Verification items for the finished model (mm, model axes). A direction names the side the tool comes from. Round coordinates to 2 decimals unless told otherwise and drop trailing zeros. Write each loop counter-clockwise with the first axis right and the second up, starting at its lowest first coordinate (ties: lowest second). Pieces come first, ordered by that corner, then holes.
from build123d import *

# Parameters (mm, degrees)
BOSS_EXTRUDE1_DEPTH = 3
BOSS_EXTRUDE2_DEPTH = 13
SKETCH4_W           = 2.5
SKETCH4_H           = 1.5
BOSS_EXTRUDE3_DEPTH = 13
SKETCH5_R           = 1.5
CUT_EXTRUDE2_DEPTH  = 10
SKETCH6_W           = 6
SKETCH6_H           = 1.5
CUT_EXTRUDE3_DEPTH  = 10


with BuildPart() as part:
    # Sketch1 → Boss-Extrude1 (new body)
    with BuildSketch(Plane(origin=(0, 0, 0), x_dir=(1, 0, 0), z_dir=(0, 1, 0))):
        Polygon((2.636620285, -0.001333349), (24.999999567, -0.001333349), (24.999999567, 6.998666651), (27.499999567, 6.998666651), (27.499999567, 0.004879765), (27.499999567, -25.613592849), (-0.500000433, -25.613592849), (0, 0), (0.136620285, 6.998666651), (2.636620285, 6.998666651), align=None)
    extrude(amount=BOSS_EXTRUDE1_DEPTH)

    # Sketch2 → Boss-Extrude2 (add)
    with BuildSketch(Plane(origin=(0, 0, 0), x_dir=(-1, 0, 0), z_dir=(0, -1, 0))):
        Polygon((-2.636620285, 6.998666651), (-0.136620285, 6.998666651), (-0.107338932, 5.498666651), (-2.636620285, 5.498666651), align=None)
    extrude(amount=BOSS_EXTRUDE2_DEPTH)

    # Sketch4 → Boss-Extrude3 (add)
    with BuildSketch(Plane(origin=(0, 0, 0), x_dir=(-1, 0, 0), z_dir=(0, -1, 0))):
        with Locations((-26.249999567, 6.248666651)):
            Rectangle(SKETCH4_W, SKETCH4_H)
    extrude(amount=BOSS_EXTRUDE3_DEPTH)

    # Sketch5 → Cut-Extrude2 (cut)
    with BuildSketch(Plane(origin=(0, 3, 0), x_dir=(1, 0, 0), z_dir=(0, 1, 0))):
        with Locations((3.669128533, -10.836145103)):
            Circle(SKETCH5_R)
        with Locations((23.902624268, -10.836145103)):
            Circle(SKETCH5_R)
    extrude(amount=-CUT_EXTRUDE2_DEPTH, mode=Mode.SUBTRACT)

    # Sketch6 → Cut-Extrude3 (cut)
    with BuildSketch(Plane(origin=(0, 3, 0), x_dir=(1, 0, 0), z_dir=(0, 1, 0))):
        with Locations((13.499999567, -21.863592849)):
            Rectangle(SKETCH6_W, SKETCH6_H)
    extrude(amount=-CUT_EXTRUDE3_DEPTH, mode=Mode.SUBTRACT)


solid = part.part
Q1. Release check for a two-part mould opening along X. For faces 1 (the flat face through (2.637, -1, -6)), 2 (the flat face through (26, -6, -5.499)), 3 (the flat face through (27.5, 0.4, 7)) record: released by +X, released by -X, zero draft, split by the parting line, or undercut.
Recorded:
face 1: undercut
face 2: zero draft
face 3: released by +X
Q2. Tool access check on faces 4 (the flat face through (10.5, 2, 22)), 5 (the flat face through (14, 1, 0.001)), 6 (the flat face through (14, 0, 13)). Record the directions out of +Z, -Z, +X, -X, +Y, -Y that give a thin tool (end or side, any length) a straight path to the whole face; none if there is none.
Recorded:
face 4: +Y, -Y
face 5: -Z, +Y, -Y
face 6: +Z, +X, -X, -Y
Q3. Material ranges on line 1 along Y through (x, z) = (14.25, 3); line 2 along Z through (x, y) = (2.25, -8), recorded low to high.
Recorded:
line 1: y = 0 to 3
line 2: z = -7 to -5.5
Q4. Sectioned sample at A-A (x = 11). Enter the section's corners in (y, z).
Recorded:
outline: (0, 0) - (3, 0) - (3, 21.11) - (0, 21.11) - close; (0, 22.61) - (3, 22.61) - (3, 25.61) - (0, 25.61) - close
Q5. Depth check by flat-ended pin: P1, Ø3, axis at x = 2, y = -3.5, coming from the +Z side; P2, Ø1.6, axis at y = 1, z = 22, coming from the -X side; P3, Ø3.5, axis at y = -1.5, z = -3.5, coming from the -X side; P4, Ø2, axis at y = -6.5, z = -5, coming from the +X side. Enter the tip coordinate at first touch or a pass-through.
Recorded:
P1: stops at z = -5.5
P2: stops at x = -0.45
P3: stops at x = 0.05
P4: stops at x = 27.5
Q6. Sectioned sample at D-D (x = 22). Enter the section's corners in (y, z).
Recorded:
outline: (0, 0) - (3, 0) - (3, 25.61) - (0, 25.61) - close
Q7. Sectioned sample at B-B (y = -11). Enter the section's corners in (x, z), plus the area to 3 significant figures.
Recorded:
outline: (0.11, -5.5) - (0.14, -7) - (2.64, -7) - (2.64, -5.5) - close; (25, -7) - (27.5, -7) - (27.5, -5.5) - (25, -5.5) - close
area: 7.52 mm2
Q8. Sectioned sample at C-C (y = 0.75). Enter the section's corners in (x, z), plus the area to 3 significant figures.
Recorded:
outline: (-0.5, 25.61) - (0.14, -7) - (2.64, -7) - (2.64, 0) - (25, 0) - (25, -7) - (27.5, -7) - (27.5, 25.61) - close; hole circle Ø3 at (3.67, 10.84); hole (10.5, 21.11) - (16.5, 21.11) - (16.5, 22.61) - (10.5, 22.61) - close; hole circle Ø3 at (23.9, 10.84)
area: 723 mm2
